The model under review builds one solid part; all positions refer to its coordinate system, in mm. Face numbers are marked on the shaded views. A direction names the side the tool comes from. Round coordinates to 2 decimals unless told otherwise and drop trailing zeros. Loops run counter-clockwise (first coordinate to the right, second up) from the corner with the lowest first, then second, coordinate; pieces in that order, holes last. Notation, with made-up numbers: (35.5, -24) -> (80.5, -24) arc R23 ccw to (80.5, 13) -> close; hole circle Ø11 at (60.25, 0). An arc over 180 degrees is marked (long way). Use a Markdown table: item, result. Add a question column.
1) Consider section B-B on y = 0.25. Give the boundary of the cut face in (x, z).
2) Consider section D-D on x = 0.75. Give the boundary of the cut face in (y, z), plus the area to 3 significant figures.
3) Consider section C-C on z = 2.5. Give the boundary of the cut face in (x, y).
4) Insertion check: pin 1 (1.5 mm diameter, centred on y = 0.5, z = 5.5, fed in from -X); pin 2 (0.9 mm diameter, centred on x = 3.5, z = 5.5, fed in from -Y); pin 3 (1 mm diameter, centred on x = 1.5, z = 2, fed in from -Y). Each pin has a flat end and moves straight along its axis. Give the tip position at first contact, or say it passes through.
5) Wall thickness on probe 1 along X at (y, z) = (1.5, -1.25); probe 2 along Y at (x, z) = (2.5, 0): over which ranges is each line inside the solid? List them lowest first.
6) Mouldability with a two-part tool opening along Z and no side actions: class the marked faces 6, 7, 8 and 9 as released by +Z, released by -Z, zero draft, split by the parting line, or undercut.
7) Consider section A-A on z = 0. Give the boundary of the cut face in (x, y), plus the area to 3 significant figures.
8) For the marked faces 1, 2, 3, 4 and 5, list the 3-axis set-ups (+Z, -Z, +X, -X, +Y, -Y) from which the entire face can be reached by the end or side of a thin tool; tool diameter is ignored.
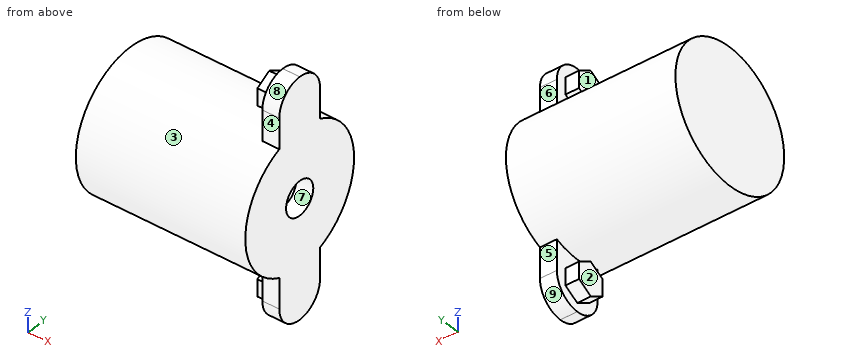
Autodesk Inventor part; units mm, degrees
ref_plane "YZ Plane" through (0, 0, 0) normal (1, 0, 0) x (0, 1, 0)
ref_plane "XZ Plane" through (0, 0, 0) normal (0, 1, 0) x (-1, 0, 0)
ref_plane "XY Plane" through (0, 0, 0) normal (0, 0, 1) x (1, 0, 0)
sketch "Sketch1" plane through (0, 0, 0) normal (0, 0, 1) x (1, 0, 0)
  line L0 (0, 0) -> (0, 4) construction
  line L1 (0, 4) -> (5, 4)
  line L2 (5, 4) -> (5, 0)
  line L3 (5, 0) -> (4, 0)
  line L4 (4, 0) -> (4, 3)
  line L5 (4, 3) -> (0, 3)
  line L6 (0, 0) -> (55.2609, 0) construction
  line L7 (0, 4) -> (-5, 4)
  line L8 (-5, 4) -> (-5, 0) construction
  line L9 (-4, 0) -> (-4, 3) construction
  line L10 (-4, 3) -> (0, 3)
  line L11 (-5, 1.5) -> (-4, 1.5)
  line L12 (-5, 1.5) -> (-5, 4)
  line L13 (-4, 1.5) -> (-4, 3)
  dimension "d0" = 1
  dimension "d1" = 3
  dimension "d2" = 0
  dimension "d3" = 1
  dimension "d4" = 5
  dimension "d5" = 1.5
revolve "Revolution1" add sketch "Sketch1" angle 360 about axis through (0, 0, 0) along (1, 0, 0)
sketch "Sketch6" plane through (5, 0, 0) normal (1, 0, 0) x (0, 0, -1)
  line L0 (0, 0) -> (-7, 0) construction
  line L1 (-7, 0) -> (-7, 1.5)
  line L2 (-7, 1.5) -> (-3.4641, 1.5)
  line L3 (0, 0) -> (0, 4) construction
  line L4 (-7, 0) -> (-7, -1.5)
  line L5 (-7, -1.5) -> (-3.4641, -1.5)
  line L6 (0, 0) -> (7, 0) construction
  line L7 (7, 0) -> (7, 1.5)
  line L8 (7, 1.5) -> (3.4641, 1.5)
  line L9 (7, 0) -> (7, -1.5)
  line L10 (7, -1.5) -> (3.4641, -1.5)
  arc A0 (-3.4641, 1.5) -> (-3.4641, -1.5) centre (0, 0) ccw construction
  arc A1 (3.4641, -1.5) -> (3.4641, 1.5) centre (0, 0) ccw construction
  line L11 (-7, -1.5) -> (-7, 1.5) construction
  line L12 (7, -1.5) -> (7, 1.5) construction
  line L13 (-7, 1.5) -> (7, 1.5)
  line L14 (-7, -1.5) -> (7, -1.5)
  dimension "d30" = 1.5
  dimension "d31" = 7
extrude "Extrusion5" add sketch "Sketch6" against normal blind 1
fillet "Fillet2" radius 1.5 4 edges at (4.5, -1.5, 7) (4.5, 1.5, 7) (4.5, -1.5, -7) (4.5, 1.5, -7)
sketch "Sketch7" plane through (4, 0, 0) normal (-1, 0, 0) x (0, 0, 1)
  arc A0 (5.5, -1.5) -> (5.5, 1.5) centre (5.5, 0) ccw
  arc A1 (-5.5, 1.5) -> (-5.5, -1.5) centre (-5.5, 0) ccw
  line L0 (-3.7081, -1.5) -> (-5.5, -1.5)
  arc A2 (-3.7081, 1.5) -> (-3.7081, -1.5) centre (0, 0) ccw
  line L1 (-5.5, 1.5) -> (-3.7081, 1.5)
  line L2 (6, 0.866) -> (6.5, 0)
  line L3 (6.5, 0) -> (6, -0.866)
  line L4 (6, -0.866) -> (5, -0.866)
  line L5 (5, -0.866) -> (4.5, 0)
  line L6 (4.5, 0) -> (5, 0.866)
  line L7 (5, 0.866) -> (6, 0.866)
  line L8 (-5, 0.866) -> (-4.5, 0)
  line L9 (-4.5, 0) -> (-5, -0.866)
  line L10 (-5, -0.866) -> (-6, -0.866)
  line L11 (-6, -0.866) -> (-6.5, 0)
  line L12 (-6.5, 0) -> (-6, 0.866)
  line L13 (-6, 0.866) -> (-5, 0.866)
  dimension "d35" = 1
extrude "Extrusion6" add sketch "Sketch7" along normal blind 0.8 contours L2 L3 L4 L5 L6 L7 | L8 L9 L10 L11 L12 L13
sketch "Sketch8" plane through (5, 0, 0) normal (1, 0, 0) x (0, 0, -1)
  arc A0 (3.7081, 1.5) -> (-3.7081, 1.5) centre (0, 0) ccw
  circle A1 centre (0, 0) radius 1
  dimension "d38" = 2
extrude "Extrusion7" cut sketch "Sketch8" against normal blind 10
sketch "Sketch9" plane through (-5, 0, 0) normal (-1, 0, 0) x (0, 0, 1)
  circle A0 centre (0, 0) radius 1.5
extrude "Extrusion8" add sketch "Sketch9" against normal blind 1
properties part number "Cylinder"
Result set:
| question | item | result |
|---|---|---|
| 1 | outline | (-5, -3.99) -> (4, -3.99) -> (4, -4.64) -> (3.2, -4.64) -> (3.2, -6.36) -> (4, -6.36) -> (4, -6.98) -> (5, -6.98) -> (5, -0.97) -> (4, -0.97) -> (4, -2.99) -> (-4, -2.99) -> (-4, 2.99) -> (4, 2.99) -> (4, 0.97) -> (5, 0.97) -> (5, 6.98) -> (4, 6.98) -> (4, 6.36) -> (3.2, 6.36) -> (3.2, 4.64) -> (4, 4.64) -> (4, 3.99) -> (-5, 3.99) -> close |
| 2 | outline | circle Ø8 at (0, 0); hole circle Ø6 at (0, 0) |
| 2 | area | 22.0 mm2 |
| 3 | outline | (-5, -3.12) -> (5, -3.12) -> (5, 3.12) -> (-5, 3.12) -> close; hole (-4, -1.66) -> (4, -1.66) -> (4, 1.66) -> (-4, 1.66) -> close |
| 4 | pin 1 | x = 3.2 |
| 4 | pin 2 | y = -0.87 |
| 4 | pin 3 | y = -3.71 |
| 5 | probe 1 | -5 to -4, 4 to 5 |
| 5 | probe 2 | -4 to -3, 3 to 4 |
| 6 | face 6 | zero draft |
| 6 | face 7 | undercut |
| 6 | face 8 | released by +Z |
| 6 | face 9 | released by -Z |
| 7 | outline | (-5, -4) -> (5, -4) -> (5, -1) -> (4, -1) -> (4, -3) -> (-4, -3) -> (-4, 3) -> (4, 3) -> (4, 1) -> (5, 1) -> (5, 4) -> (-5, 4) -> close |
| 7 | area | 30.0 mm2 |
| 8 | face 1 | +Z, -X, +Y, -Y |
| 8 | face 2 | -Z, -X, +Y, -Y |
| 8 | face 3 | -X |
| 8 | face 4 | +Z, +X, -X, -Y |
| 8 | face 5 | -Z, +X, -X, +Y |
